The listing builds one solid part. Answer for the finished solid, in the listing's coordinates (mm). A direction names the side the tool comes from. Coordinates: 2 decimals unless noted, no trailing zeros. Order: outer loops, then holes, each group sorted by start corner. A loop starts at its lowest first (then second) coordinate and runs counter-clockwise, first axis right, second up. Notation, with made-up numbers: (-30.5, 68) -> (27.5, 68) arc R26 cw to (27.5, 92) -> close; hole circle Ø10 at (34, 40). An arc over 180 degrees is marked (long way). Return JSON: item names as keys, results as strings.
from build123d import *

# Parameters (mm, degrees)
F0_W     = 11.176
F0_H     = 11.176
F1_DEPTH = 13.97
F2_SIZE  = 1
F3_R     = 1.9939
F4_DEPTH = 15


with BuildPart() as f1:
    # F0 (on Top) → F1 (new body)
    with BuildSketch(Plane.XY):
        Rectangle(F0_W, F0_H)
    extrude(amount=F1_DEPTH)

    # F2
    f2_edges = [f1.edges().sort_by_distance(p)[0] for p in [
        (5.588, 5.588, 6.985),
        (5.588, -5.588, 6.985),
        (-5.588, -5.588, 6.985),
        (-5.588, 5.588, 6.985),
    ]]
    chamfer(f2_edges, length=F2_SIZE)

    # F3 (on face) → F4 (join)
    with BuildSketch(Plane(origin=(0, 0, 0), x_dir=(1, 0, 0), z_dir=(0, 0, -1))):
        Circle(F3_R)
    extrude(amount=F4_DEPTH)


solid = f1.part
1. The part is cut by section D-D on x = 3.25. Give the vertices of the cut face in (y, z), and give its area (3 significant figures).
Answer block:
{"outline": "(-5.59, 0) -> (5.59, 0) -> (5.59, 13.97) -> (-5.59, 13.97) -> close", "area": "156 mm2"}
2. Each of these flat-tipped pins is pushed along its axis until it touches: pin 1 Ø5 at (y, z) = (-3, -8.5) entering from -X; pin 2 Ø1.5 at (y, z) = (-1, -11) entering from -X; pin 3 Ø1.5 at (x, y) = (2.5, -1.5) entering from -Z. Where does it stop, or does it pass through?
Answer block:
{"pin 1": "stops at x = -1.93", "pin 2": "stops at x = -1.98", "pin 3": "stops at z = 0"}
3. For faces 1 (the face through (-5.081, 5.095, 6.887)), 2 (the face through (2.4, 0.1, 0)), determine the directions among +Z, -Z, +X, -X, +Y, -Y from which every point of the face is accessible in a straight line to the end or side of a thin tool.
Answer block:
{"face 1": "+Z, -Z, -X, +Y", "face 2": "-Z"}
4. Consider line 1 (Z direction, x = 4.75, y = 1.75); line 2 (X direction, y = 0, z = -10.5); line 3 (Y direction, x = 0.25, z = -2). Determine where each line is inside the solid, lowest interval first. Write a range as from..to.
Answer block:
{"line 1": "z = 0..13.97", "line 2": "x = -1.99..1.99", "line 3": "y = -1.98..1.98"}
5. The part is cut by section C-C on z = -7.75. Give the vertices of the cut face in (x, y).
Answer block:
{"outline": "circle Ø3.99 at (0, 0)"}
6. The part is cut by section A-A on x = 0. Give the vertices of the cut face in (y, z), and give its area (3 significant figures).
Answer block:
{"outline": "(-5.59, 0) -> (-1.99, 0) -> (-1.99, -15) -> (1.99, -15) -> (1.99, 0) -> (5.59, 0) -> (5.59, 13.97) -> (-5.59, 13.97) -> close", "area": "216 mm2"}
